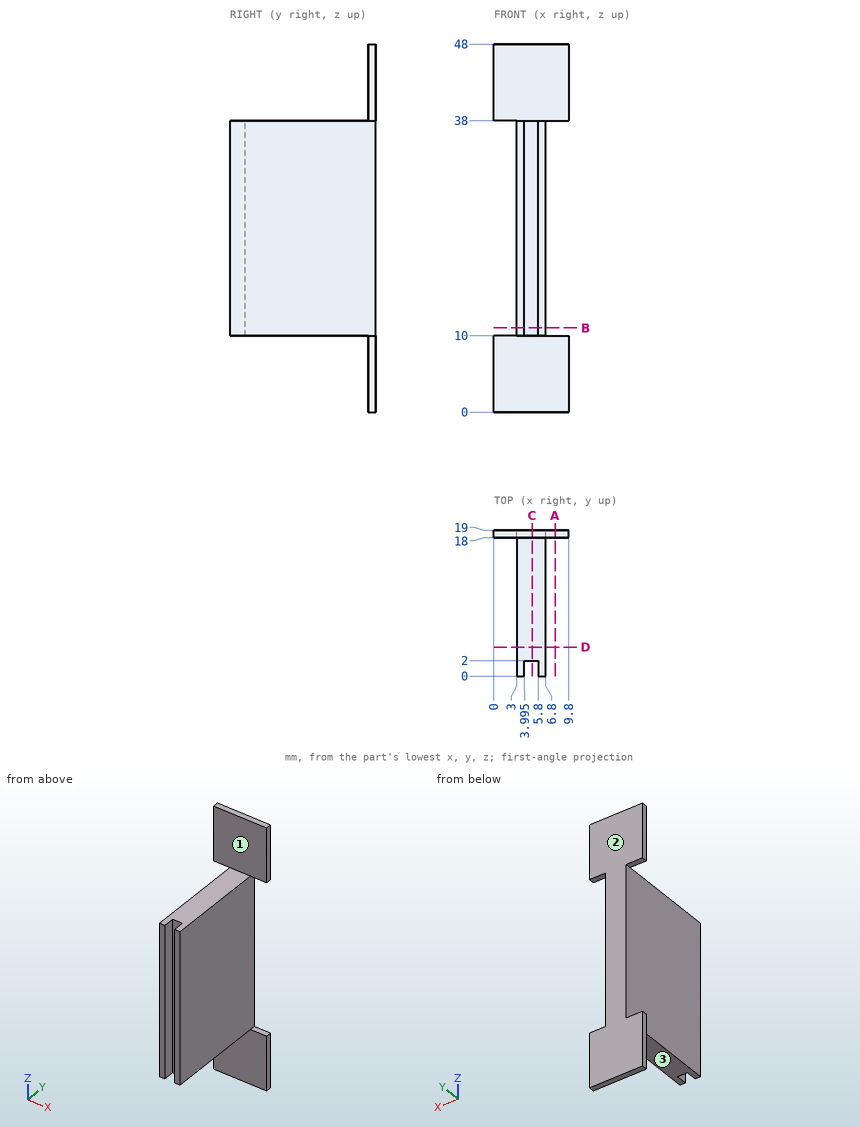
Can you work these out from the drawing? Everything is in mm from the part's minimum corner. A direction names the side the tool comes from. Give positions to 0.01 mm unless a question says otherwise; leave off trailing zeros. Loops run counter-clockwise (first coordinate to the right, second up) from the corner with the lowest first, then second, coordinate; pieces in that order, holes last. Notation, with made-up numbers: (-36, -12.5) -> (-19, -12.5) arc R16 cw to (-19, 0.5) -> close; hole circle Ø9 at (41.25, 57). An arc over 180 degrees is marked (long way). Return JSON: item names as keys, results as strings.
Q1. I want a section at C-C, the plane x = 5. List the corners of the cut face in (y, z) for me, then the cut area to 3 significant figures.
Checks:
{"outline": "(2, 10) -> (18, 10) -> (18, 0) -> (19, 0) -> (19, 48) -> (18, 48) -> (18, 38) -> (2, 38) -> close", "area": "496 mm2"}
Q2. For pin 1 Ø1.9 at (x, y) = (4, 5.5) entering from +Z; pin 2 Ø3 at (y, z) = (11, 30) entering from -X; pin 3 Ø0.6 at (y, z) = (1, 27.5) entering from +X, each with a flat end and sliding along its axis, tell me the tip position at first contact or that it passes through.
Checks:
{"pin 1": "stops at z = 38", "pin 2": "stops at x = 3", "pin 3": "stops at x = 6.8"}
Q3. I want a section at D-D, the plane y = 3.75. List the corners of the cut face in (x, z) for me.
Checks:
{"outline": "(3, 10) -> (6.8, 10) -> (6.8, 38) -> (3, 38) -> close"}
Q4. I need wall thicknesses on probe 1 along X at (y, z) = (1.5, 21.5) (1 decimal); probe 2 along Z at (x, y) = (3.25, 8.5); probe 3 along X at (y, z) = (18, 19.5). Which ranges of each line are inside material? Lowest first, please.
Checks:
{"probe 1": "x = 3 to 4, 5.8 to 6.8", "probe 2": "z = 10 to 38", "probe 3": "x = 3 to 6.8"}
Q5. On a 3-axis mill with a long thin cutter (end or side, diameter ignored), from which of +Z, -Z, +X, -X, +Y, -Y can I reach the whole of each face in a straight line? I mean the marked faces 1, 2 and 3. Say none if no direction works.
Checks:
{"face 1": "+Z, +X, -X, -Y", "face 2": "+Z, -Z, +X, -X, +Y", "face 3": "-Z, +X, -X, -Y"}
Q6. I want a section at B-B, the plane z = 11. List the corners of the cut face in (x, y) for me (1 decimal).
Checks:
{"outline": "(3, 0) -> (4, 0) -> (4, 2) -> (5.8, 2) -> (5.8, 0) -> (6.8, 0) -> (6.8, 19) -> (3, 19) -> close"}
Q7. I want a section at A-A, the plane x = 8. List the corners of the cut face in (y, z) for me, then the cut area to 3 significant figures.
Checks:
{"outline": "(18, 0) -> (19, 0) -> (19, 10) -> (18, 10) -> close; (18, 38) -> (19, 38) -> (19, 48) -> (18, 48) -> close", "area": "20.0 mm2"}
